Part model, mm, in its own coordinate system. A direction names the side the tool comes from. Round coordinates to 2 decimals unless told otherwise and drop trailing zeros. Order: outer loops, then holes, each group sorted by start corner. A loop starts at its lowest first (then second) coordinate and runs counter-clockwise, first axis right, second up. Notation, with made-up numbers: (18, 43.5) - (22, 43.5) arc R24 ccw to (22, 67.5) - close; hole circle Ø9 at (82, 68). An arc over 180 degrees is marked (long way). Answer as a JSON object with one key per item and string values.
Autodesk Inventor part; units mm, degrees
ref_plane "YZ Plane" through (0, 0, 0) normal (1, 0, 0) x (0, 1, 0)
ref_plane "XZ Plane" through (0, 0, 0) normal (0, 1, 0) x (-1, 0, 0)
ref_plane "XY Plane" through (0, 0, 0) normal (0, 0, 1) x (1, 0, 0)
sketch "Sketch1" plane through (0, 0, 0) normal (0, 0, 1) x (1, 0, 0)
  line L0 (0, 0) -> (310, 0)
  line L1 (310, 0) -> (310, 50)
  line L2 (310, 50) -> (0, 50)
  line L3 (0, 50) -> (0, 0)
  dimension "d0" = 310
  dimension "d1" = 50
extrude "Extrusion1" add sketch "Sketch1" along normal blind 18.55
sketch "Sketch2" plane through (0, 0, 18.55) normal (0, 0, 1) x (1, 0, 0)
  line L0 (130, 34.3) -> (180, 34.3)
  line L1 (180, 34.3) -> (180, 15.7)
  line L2 (180, 15.7) -> (130, 15.7)
  line L3 (130, 15.7) -> (130, 34.3)
  line L4 (130, 25) -> (0, 25) construction
  line L5 (0, 50) -> (0, 0)
  line L6 (180, 25) -> (310, 25) construction
  line L7 (310, 0) -> (310, 50)
  dimension "d4" = 18.6
  dimension "d5" = 50
extrude "Extrusion2" cut sketch "Sketch2" against normal blind 20
properties part number "mobile_table_bottom"
Item 1: Drop a flat-ended pin along its axis: P1, Ø10, axis at x = 91, y = 21, coming from the -Z side. Give the stop position or say it passes through.
Taken from the geometry:
{"P1": "z = 0"}
Item 2: Tool access for faces 1 (the flat face through (153, 0, 9)), 2 (the flat face through (130, 25, 9)): list every direction of +Z, -Z, +X, -X, +Y, -Y with a clear straight run to the whole face (end or side of a thin tool).
Taken from the geometry:
{"face 1": "+Z, -Z, +X, -X, -Y", "face 2": "+Z, -Z"}
Item 3: Two-plate mould, pull along X, no slides. Class faces 3 (the flat face through (155, 34.3, 9)), 4 (the flat face through (310, 25, 9)), 5 (the flat face through (153, 36, 18.55)), 6 (the flat face through (0, 25, 9)): pulls with the +X half, pulls with the -X half, needs draft (parallel to the pull), parting line crosses it, or undercut.
Taken from the geometry:
{"face 3": "undercut", "face 4": "pulls with the +X half", "face 5": "needs draft", "face 6": "pulls with the -X half"}
Item 4: Cut at C-C (x = 170). Write the cut outline in (y, z), plus the area to 3 significant figures.
Taken from the geometry:
{"outline": "(0, 0) - (15.7, 0) - (15.7, 18.55) - (0, 18.55) - close; (34.3, 0) - (50, 0) - (50, 18.55) - (34.3, 18.55) - close", "area": "582 mm2"}
Item 5: Probe L1, parallel to Y at x = 176, z = 4; L2, parallel to X at y = 29, z = 5.5. List the from-to ranges inside material, lowest first. Write a range as from..to.
Taken from the geometry:
{"L1": "0..15.7, 34.3..50", "L2": "0..130, 180..310"}
Item 6: Cut at B-B (y = 22.5). Write the cut outline in (x, z).
Taken from the geometry:
{"outline": "(0, 0) - (130, 0) - (130, 18.55) - (0, 18.55) - close; (180, 0) - (310, 0) - (310, 18.55) - (180, 18.55) - close"}
Item 7: Cut at A-A (z = 11.25). Write the cut outline in (x, y).
Taken from the geometry:
{"outline": "(0, 0) - (310, 0) - (310, 50) - (0, 50) - close; hole (130, 15.7) - (180, 15.7) - (180, 34.3) - (130, 34.3) - close"}
